Geometry: final body of the model. Coordinates: model frame, mm. Give positions to 0.01 mm unless a question says otherwise; leave off trailing zeros. Loops run counter-clockwise (first coordinate to the right, second up) from the corner with the lowest first, then second, coordinate; pieces in that order, holes last. Notation, with made-up numbers: (88, -21.75) - (93, -21.75) arc R24 cw to (93, -2.75) - close; hole circle Ø2 at (-34, 79). An arc over 180 degrees is marked (long way). Answer in a Markdown table with one row per item.
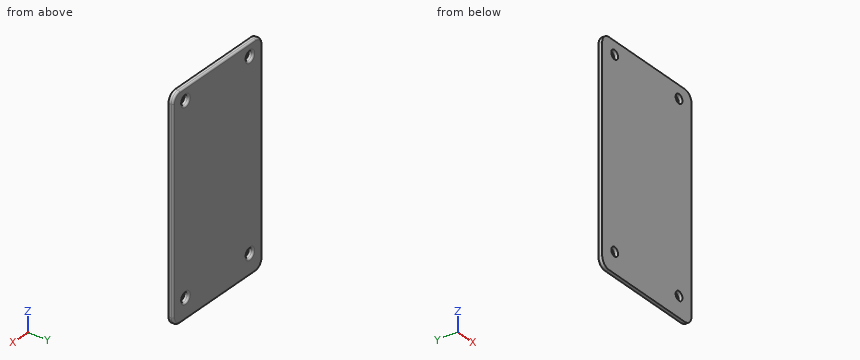
from build123d import *

# Parameters (mm, degrees)
SKETCH1_W           = 33
SKETCH1_H           = 60
BOSS_EXTRUDE1_DEPTH = 1.27
CUT_EXTRUDE1_REACH  = 3.27
SKETCH2_R           = 1.245715159
SKETCH2_R_2         = 1.25
FILLET1_R           = 2.50000008
FILLET2_R           = 0.508


with BuildPart() as part:
    # Sketch1 → Boss-Extrude1 (new body)
    with BuildSketch(Plane(origin=(0, 0, 0), x_dir=(1, 0, 0), z_dir=(0, 1, 0))):
        with Locations((16.989591658, -21.38828823)):
            Rectangle(SKETCH1_W, SKETCH1_H)
    extrude(amount=BOSS_EXTRUDE1_DEPTH)

    # Sketch2 → Cut-Extrude1 (cut, up to next)
    with BuildSketch(Plane(origin=(0, 1.27, 0), x_dir=(1, 0, 0), z_dir=(0, 1, 0)), mode=Mode.PRIVATE) as cut_extrude1_sk1:
        with Locations((5.093876499, 2.96171177)):
            Circle(SKETCH2_R)
    cut_extrude1_tool1 = extrude(cut_extrude1_sk1.sketch, amount=-CUT_EXTRUDE1_REACH, mode=Mode.PRIVATE) & part.part
    add(cut_extrude1_tool1.solids().sort_by_distance((5.093876, 1.27, -2.961712))[0], mode=Mode.SUBTRACT)
    # Sketch2 → Cut-Extrude1 (cut, up to next)
    with BuildSketch(Plane(origin=(0, 1.27, 0), x_dir=(1, 0, 0), z_dir=(0, 1, 0)), mode=Mode.PRIVATE) as cut_extrude1_sk2:
        with Locations((28.889591658, 2.96171177)):
            Circle(SKETCH2_R_2)
    cut_extrude1_tool2 = extrude(cut_extrude1_sk2.sketch, amount=-CUT_EXTRUDE1_REACH, mode=Mode.PRIVATE) & part.part
    add(cut_extrude1_tool2.solids().sort_by_distance((28.889592, 1.27, -2.961712))[0], mode=Mode.SUBTRACT)
    # Sketch2 → Cut-Extrude1 (cut, up to next)
    with BuildSketch(Plane(origin=(0, 1.27, 0), x_dir=(1, 0, 0), z_dir=(0, 1, 0)), mode=Mode.PRIVATE) as cut_extrude1_sk3:
        with Locations((5.089591658, -47.83828823)):
            Circle(SKETCH2_R_2)
    cut_extrude1_tool3 = extrude(cut_extrude1_sk3.sketch, amount=-CUT_EXTRUDE1_REACH, mode=Mode.PRIVATE) & part.part
    add(cut_extrude1_tool3.solids().sort_by_distance((5.089592, 1.27, 47.838288))[0], mode=Mode.SUBTRACT)
    # Sketch2 → Cut-Extrude1 (cut, up to next)
    with BuildSketch(Plane(origin=(0, 1.27, 0), x_dir=(1, 0, 0), z_dir=(0, 1, 0)), mode=Mode.PRIVATE) as cut_extrude1_sk4:
        with Locations((28.889591658, -47.83828823)):
            Circle(SKETCH2_R_2)
    cut_extrude1_tool4 = extrude(cut_extrude1_sk4.sketch, amount=-CUT_EXTRUDE1_REACH, mode=Mode.PRIVATE) & part.part
    add(cut_extrude1_tool4.solids().sort_by_distance((28.889592, 1.27, 47.838288))[0], mode=Mode.SUBTRACT)

    # Fillet1
    fillet1_edges = [part.edges().sort_by_distance(p)[0] for p in [
        (0.489591658, 0.635, -8.61171177),
        (33.489591658, 0.635, -8.61171177),
        (33.489591658, 0.635, 51.38828823),
        (0.489591658, 0.635, 51.38828823),
    ]]
    fillet(fillet1_edges, radius=FILLET1_R)

    # Fillet2
    fillet2_edges = [part.edges().sort_by_distance(p)[0] for p in [
        (27.639591658, 1.27, -2.96171177),
        (3.839591658, 1.27, 47.83828823),
        (27.639591658, 1.27, 47.83828823),
        (3.84816134, 1.27, -2.96171177),
        (33.489591658, 1.27, 21.38828823),
        (16.989591658, 1.27, 51.38828823),
        (0.489591658, 1.27, 21.38828823),
        (16.989591658, 1.27, -8.61171177),
        (32.757358588, 1.27, -7.8794787),
        (1.221824728, 1.27, -7.8794787),
        (1.221824728, 1.27, 50.65605516),
        (32.757358588, 1.27, 50.65605516),
    ]]
    fillet(fillet2_edges, radius=FILLET2_R)


solid = part.part
Q1. First-contact query: pin 1 (2 mm diameter, centred on x = 5.09, z = 47.84, fed in from -Y). Flat tip, straight axial feed; report the tip coordinate or a pass-through.
Check values:
| item | result |
|---|---|
| pin 1 | through |
Q2. Cut plane A-A (y = 1). Output: boundary loops of the cut face in (x, z).
Check values:
| item | result |
|---|---|
| outline | (0.55, -6.11) arc R2.44 ccw to (2.99, -8.55) - (30.99, -8.55) arc R2.44 ccw to (33.43, -6.11) - (33.43, 48.89) arc R2.44 ccw to (30.99, 51.33) - (2.99, 51.33) arc R2.44 ccw to (0.55, 48.89) - close; hole circle Ø2.62 at (5.09, 47.84); hole circle Ø2.61 at (5.09, -2.96); hole circle Ø2.62 at (28.89, -2.96); hole circle Ø2.62 at (28.89, 47.84) |
Q3. Material intervals for line 1 along Z through (x, y) = (5, 0.55); line 2 along Z through (x, y) = (28.5, 0.5); line 3 along X through (y, z) = (0.7, -2), sorted ascending.
Check values:
| item | result |
|---|---|
| line 1 | -8.61 to -4.2, -1.72 to 46.59, 49.09 to 51.39 |
| line 2 | -8.61 to -4.15, -1.77 to 46.65, 49.03 to 51.39 |
| line 3 | 0.49 to 4.3, 5.89 to 28.09, 29.69 to 33.49 |
